```python
from build123d import *

# Parameters (mm, degrees)
BOSS_EXTRUDE1_DEPTH = 4
SKETCH2_R           = 1
BOSS_EXTRUDE2_DEPTH = 1


with BuildPart() as part:
    # Sketch1 → Boss-Extrude1 (new body)
    with BuildSketch(Plane(origin=(0, 0, 0), x_dir=(0, 0, -1), z_dir=(1, 0, 0))):
        with BuildLine():
            Line((0, 7), (-16.2, 4.5))
            ThreePointArc((-16.2, 4.5), (-18.456321812, 0.070210727), (-16.5, -4.5))
            Line((-16.5, -4.5), (0, -7))
            Line((0, -7), (16.5, -4.5))
            ThreePointArc((16.5, -4.5), (18.456321812, 0.070210727), (16.2, 4.5))
            Line((16.2, 4.5), (0, 7))
        make_face()
        with BuildLine():
            Line((0, 3.7), (-15.2, 1.9))
            ThreePointArc((-15.2, 1.9), (-16.123290742, 0), (-15.2, -1.9))
            Line((-15.2, -1.9), (0, -3.7))
            Line((0, -3.7), (15.2, -1.9))
            ThreePointArc((15.2, -1.9), (16.123290742, 0), (15.2, 1.9))
            Line((15.2, 1.9), (0, 3.7))
        make_face(mode=Mode.SUBTRACT)
    extrude(amount=BOSS_EXTRUDE1_DEPTH)

    # Sketch2 → Boss-Extrude2 (add)
    with BuildSketch(Plane(origin=(0, 0, 0), x_dir=(0, 0, -1), z_dir=(1, 0, 0))):
        with BuildLine():
            Line((0, 7), (-16.2, 4.5))
            ThreePointArc((-16.2, 4.5), (-18.456321812, 0.070210727), (-16.5, -4.5))
            Line((-16.5, -4.5), (0, -7))
            Line((0, -7), (16.5, -4.5))
            ThreePointArc((16.5, -4.5), (18.456321812, 0.070210727), (16.2, 4.5))
            Line((16.2, 4.5), (0, 7))
        make_face()
        Circle(SKETCH2_R, mode=Mode.SUBTRACT)
    extrude(amount=-BOSS_EXTRUDE2_DEPTH)


solid = part.part
```
Verification items for the finished model (mm, model axes). A direction names the side the tool comes from. Coordinates: 2 decimals unless noted, no trailing zeros. Loops run counter-clockwise (first coordinate to the right, second up) from the corner with the lowest first, then second, coordinate; pieces in that order, holes last. Notation, with made-up numbers: (69, 40.5) - (98, 40.5) arc R18 cw to (98, 54.5) - close; hole circle Ø10 at (1.25, 58). An arc over 180 degrees is marked (long way). Put each result on its own line as item: value.
Item 1: Section check D-D (y = 5.75). Enter the section's corners in (x, z), then the cut area to 3 significant figures.
Conclusion:
outline: (-1, -8.1) - (4, -8.1) - (4, 8.1) - (-1, 8.1) - close
area: 81.0 mm2
Item 2: Draft check along Z on faces 3 (the face through (1.972, -0.031, -16.123)), 4 (the face through (1.54, -5.77, -8.13)), 5 (the face through (1.972, -2.813, -7.494)), 6 (the face through (1.54, -5.73, 8.37)). Enter one of: pulls with the +Z half, pulls with the -Z half, needs draft (parallel to the pull), parting line crosses it, or undercut.
Conclusion:
face 3: undercut
face 4: pulls with the -Z half
face 5: undercut
face 6: pulls with the +Z half
Item 3: Section check C-C (z = -10.5). Enter the section's corners in (x, y), then the cut area to 3 significant figures.
Conclusion:
outline: (-1, -5.41) - (4, -5.41) - (4, -2.46) - (0, -2.46) - (0, 2.46) - (4, 2.46) - (4, 5.38) - (-1, 5.38) - close
area: 34.3 mm2
Item 4: Section check A-A (x = 1.35). Enter the section's corners in (y, z), then the cut area to 3 significant figures.
Conclusion:
outline: (-7, 0) - (-4.5, -16.5) arc R5.86 ccw to (4.5, -16.2) - (7, 0) - (4.5, 16.2) arc R5.86 ccw to (-4.5, 16.5) - close; hole (-3.7, 0) - (-1.9, -15.2) arc R2.42 ccw to (1.9, -15.2) - (3.7, 0) - (1.9, 15.2) arc R2.42 ccw to (-1.9, 15.2) - close
area: 227 mm2
Item 5: Section check B-B (y = 0). Enter the section's corners in (x, z), then the cut area to 3 significant figures.
Conclusion:
outline: (-1, -18.46) - (4, -18.46) - (4, -16.12) - (0, -16.12) - (0, -1) - (-1, -1) - close; (-1, 1) - (0, 1) - (0, 16.12) - (4, 16.12) - (4, 18.46) - (-1, 18.46) - close
area: 53.6 mm2
Item 6: Set-up check for faces 1 (the face through (1.972, 0.031, 16.123)), 2 (the face through (1.535, 5.768, 7.987)): record each of +Z, -Z, +X, -X, +Y, -Y from which the full face is reachable in a straight line by a thin tool's end or side.
Conclusion:
face 1: +X
face 2: +Z, +X, -X, +Y
Item 7: Gauge pin test, flat ends, axial feed: pin 1 Ø1 at (x, y) = (1, 2) entering from +Z; pin 2 Ø3 at (x, z) = (1.5, 10) entering from -Y. Record the tip position at first contact, or that the pin passes through.
Conclusion:
pin 1: stops at z = 18.23
pin 2: stops at y = -5.71
Item 8: Scan lines: line 1 along Y through (x, z) = (-0.25, 0); line 2 along Y through (x, z) = (0.15, -5); line 3 along Z through (x, y) = (3.3, 4.25). Record each from-to range of solid material in increasing order.
Conclusion:
line 1: y = -7 to -1, 1 to 7
line 2: y = -6.24 to -3.11, 3.11 to 6.23
line 3: z = -16.5 to 16.5
